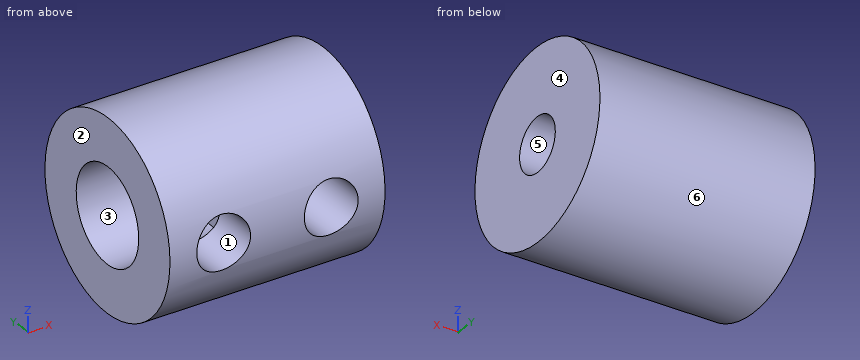
```python
from build123d import *

# Parameters (mm, degrees)
SKETCH1_W         = 25.4
SKETCH1_H         = 11.1125
HOLE1_D           = 6.35
HOLE1_CBORE_D     = 11.1125
HOLE1_CBORE_DEPTH = 12.7
SKETCH4_W         = 3.175
SKETCH4_H         = 11.1125
HOLE3_D           = 6.35
HOLE3_DEPTH       = 6.552753399


with BuildPart() as part:
    # Sketch1 → Revolve1 (revolve)
    with BuildSketch(Plane.XY, mode=Mode.PRIVATE) as revolve1_sk:
        with Locations((0, 5.55625)):
            Rectangle(SKETCH1_W, SKETCH1_H)
    revolve(revolve1_sk.sketch.rotate(Axis((-12.7, 0, 0), (1, 0, 0)), 270), axis=Axis((-12.7, 0, 0), (1, 0, 0)))

    # Hole1 (through all)
    with Locations(Plane.ZY.offset(12.7)):
        with Locations((0, 0)):
            CounterBoreHole(HOLE1_D / 2, HOLE1_CBORE_D / 2, HOLE1_CBORE_DEPTH)

    # Sketch4 → Hole2 (revolve, cut)
    with BuildSketch(Plane(origin=(6.35, 0, 0), x_dir=(0, 0, 1), z_dir=(1, 0, 0))):
        with Locations((1.5875, 5.55625)):
            Rectangle(SKETCH4_W, SKETCH4_H)
    revolve(axis=Axis((6.35, -110, 0), (0, 1, 0)), mode=Mode.SUBTRACT)

    # Hole3
    with Locations(Plane(origin=(0, -4.559746601, 0), x_dir=(1, 0, 0), z_dir=(0, 1, 0))):
        with Locations((-6.35, 0)):
            Hole(HOLE3_D / 2, depth=HOLE3_DEPTH)


solid = part.part
```
The listing builds one solid part. Answer for the finished solid, in the listing's coordinates (mm). Face numbers are marked on the shaded views. A direction names the side the tool comes from. Give positions to 0.01 mm unless a question says otherwise; leave off trailing zeros. Order: outer loops, then holes, each group sorted by start corner. A loop starts at its lowest first (then second) coordinate and runs counter-clockwise, first axis right, second up. Notation, with made-up numbers: (32, 28.5) -> (79, 28.5) arc R6 ccw to (79, 37.5) -> close; hole circle Ø5 at (78, 14). An arc over 180 degrees is marked (long way). One line per item, written item: value.
1) Find section B-B, the plane y = -1. Determine the outline of the cut face in (x, z) (3 decimals).
Reported:
outline: (-12.7, -11.067) -> (12.7, -11.067) -> (12.7, -3.013) -> (7.35, -3.013) arc R3.175 cw to (5.35, -3.013) -> (0, -3.013) -> (0, -5.466) -> (-12.7, -5.466) -> close; (-12.7, 5.466) -> (0, 5.466) -> (0, 3.013) -> (5.35, 3.013) arc R3.175 cw to (7.35, 3.013) -> (12.7, 3.013) -> (12.7, 11.067) -> (-12.7, 11.067) -> close
2) A tool of negligible diameter and unlimited length cuts with its end or side. For the marked faces 1, 2 and 3, from which of +Z, -Z, +X, -X, +Y, -Y can it reach the whole face along a straight path? Write none if from no direction.
Reported:
face 1: -Y
face 2: +Z, -Z, -X, +Y, -Y
face 3: -X
3) Find section D-D, the plane y = 4.25. Determine the outline of the cut face in (x, z).
Reported:
outline: (-12.7, -10.27) -> (12.7, -10.27) -> (12.7, 10.27) -> (-12.7, 10.27) -> (-12.7, 3.58) -> (0, 3.58) -> (0, -3.58) -> (-12.7, -3.58) -> close
4) Determine the mould class of the marked faces 4, 5 and 6 for opening direction Z: pulls with the +Z half, pulls with the -Z half, needs draft (parallel to the pull), parting line crosses it, or undercut.
Reported:
face 4: needs draft
face 5: undercut
face 6: parting line crosses it
5) Flat-ended cylindrical pins translate along their axes: P1, Ø8.5, axis at y = 0, z = 0, coming from the -X side; P2, Ø4, axis at x = 5.5, y = -5, coming from the -Z side; P3, Ø3, axis at x = 7.5, z = -7.5, coming from the -Y side. Find the tip coordinate at first contact, or state that the pin passes through.
Reported:
P1: stops at x = 0
P2: stops at z = -10.7
P3: stops at y = -9.35
6) Find the intervals of material crossed by line 1 (X direction, y = 4, z = 0.5); line 2 (Y direction, x = 9.75, z = 0) (1 decimal); line 3 (Y direction, x = -5.5, z = 0), in increasing order.
Reported:
line 1: x = 0 to 12.7
line 2: y = -11.1 to -3.2, 3.2 to 11.1
line 3: y = 5.56 to 11.11
7) Find section A-A, the plane z = 1. Determine the outline of the cut face in (x, y).
Reported:
outline: (-12.7, -11.07) -> (-9.36, -11.07) -> (-9.36, -5.47) -> (-12.7, -5.47) -> close; (-12.7, 5.47) -> (0, 5.47) -> (0, 3.01) -> (12.7, 3.01) -> (12.7, 11.07) -> (-12.7, 11.07) -> close; (-3.34, -11.07) -> (3.34, -11.07) -> (3.34, -3.01) -> (0, -3.01) -> (0, -5.47) -> (-3.34, -5.47) -> close; (9.36, -11.07) -> (12.7, -11.07) -> (12.7, -3.01) -> (9.36, -3.01) -> close
